Input: dimensioned drawing with shaded views. Units: mm. Origin: part minimum x, y, z. Round coordinates to 2 decimals unless told otherwise and drop trailing zeros. Loops run counter-clockwise (first coordinate to the right, second up) from the corner with the lowest first, then second, coordinate; pieces in that order, holes last.
1) Ray query, line 1 along X through (y, z) = (3.85, 1.4); line 2 along Z through (x, y) = (31, 2.45); line 3 along X through (y, z) = (0.3, 3.1). Return the intervals inside material, ascending.
2) Section B-B, the plane y = 2.5. State how many separate pieces and enclosed holes the cut face has, and give its area (3 significant figures).
3) Section A-A, the plane x = 32.5. Return loops of the section in (y, z).
4) Section D-D, the plane x = 25.5. Return loops of the section in (y, z).
5) First-contact query: pin 1 (0.6 mm diameter, centred on y = 3.5, z = 2.5, fed in from +X); pin 2 (1.5 mm diameter, centred on x = 26, y = 1.5, fed in from -Z). Flat tips, straight axial feed; report the tip coordinate or a pass-through.
6) Draft query along X for the marked faces 1, 2 and 3. Return one class per face: pulls with the +X half, pulls with the -X half, needs draft (parallel to the pull), parting line crosses it, or undercut.
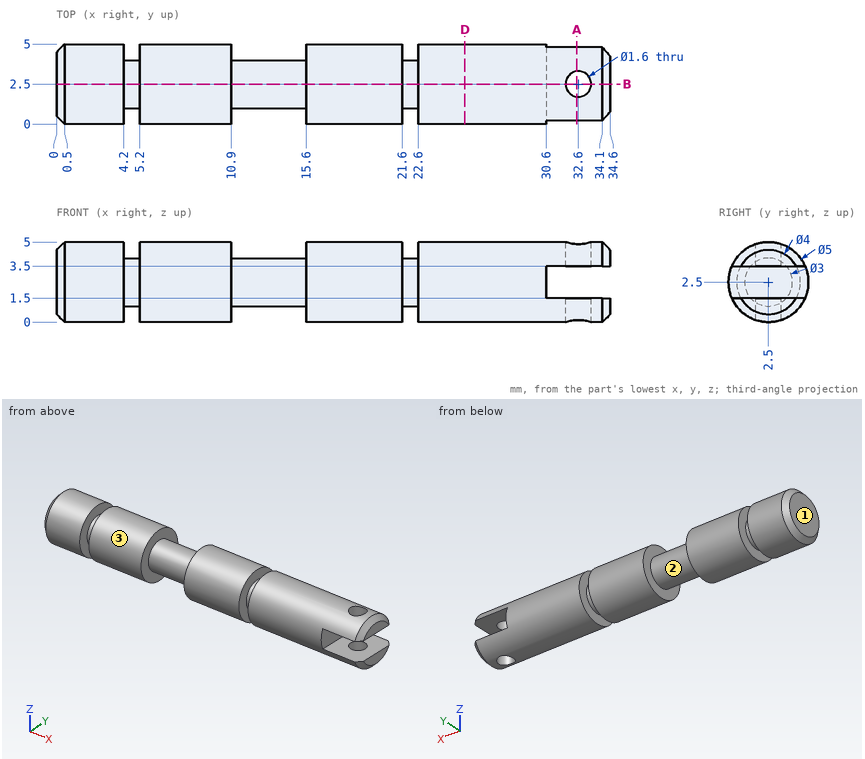
Final values:
1. line 1: x = 0 to 4.2, 5.2 to 10.9, 15.6 to 21.6, 22.6 to 34.6
1. line 2: z = 0 to 1.5, 3.5 to 5
1. line 3: x = 0.28 to 4.2, 5.2 to 10.9, 15.6 to 21.6, 22.6 to 30.6
2. separate pieces: 3
2. enclosed holes: 0
2. area: 146 mm2
3. outline: (0.21, 1.5) arc R2.5 ccw to (1.71, 0.13) - (1.71, 1.5) - close; (0.21, 3.5) - (1.71, 3.5) - (1.71, 4.87) arc R2.5 ccw to start; (3.29, 0.13) arc R2.5 ccw to (4.79, 1.5) - (3.29, 1.5) - close; (3.29, 3.5) - (4.79, 3.5) arc R2.5 ccw to (3.29, 4.87) - close
4. outline: circle Ø5 at (2.5, 2.5)
5. pin 1: stops at x = 30.6
5. pin 2: stops at z = 0.01
6. face 1: pulls with the -X half
6. face 2: undercut
6. face 3: needs draft
